For this review, take the finished solid that the model builds, in its own axes (mm). Round coordinates to 2 decimals unless told otherwise and drop trailing zeros. Loops run counter-clockwise (first coordinate to the right, second up) from the corner with the lowest first, then second, coordinate; pieces in that order, holes last. Notation, with made-up numbers: (-30.75, 60) -> (-11.75, 60) arc R29 ccw to (-11.75, 96) -> close; hole circle Ø5 at (65, -16.5). An arc over 180 degrees is marked (long way). Use one line per item in the form item = value. Start each with the question number.
from build123d import *

# Parameters (mm, degrees)
SKETCH_1_W          = 271
SKETCH_1_H          = 420.5
EXTRUDE_1_DEPTH     = 4
SKETCH_2_R          = 2.1
CUT_EXTRUDE_1_DEPTH = 251.162572141
EXTRUDE_2_DEPTH     = 4
FILLET_2_R          = 10
SKETCH_7_R          = 1.6
CUT_EXTRUDE_4_DEPTH = 261.756231949
SKETCH_8_W          = 88
SKETCH_8_H          = 60
EXTRUDE_3_DEPTH     = 4
FILLET_3_R          = 10
SKETCH_9_R          = 2.1
CUT_EXTRUDE_5_DEPTH = 303.34303779
SKETCH_10_R         = 2.6
CUT_EXTRUDE_6_DEPTH = 4
SKETCH_12_W         = 271
SKETCH_12_H         = 62.828427
EXTRUDE_4_DEPTH     = 4
FILLET_4_R          = 10


with BuildPart() as part:
    # 草图1 → 凸台-拉伸1 (new body)
    with BuildSketch(Plane(origin=(0, 0, 0), x_dir=(1, 0, 0), z_dir=(0, 1, 0))):
        Rectangle(SKETCH_1_W, SKETCH_1_H)
    extrude(amount=EXTRUDE_1_DEPTH)

    # 草图2 → 切除-拉伸1 (cut, through all)
    with BuildSketch(Plane(origin=(0, 4, 0), x_dir=(1, 0, 0), z_dir=(0, 1, 0))):
        with Locations(Location((112, 195.75, 0), (0, 0, 270))):
            Circle(SKETCH_2_R)
        with Locations(Location((128, 195.75, 0), (0, 0, 270))):
            Circle(SKETCH_2_R)
        with Locations(Location((112, 163.75, 0), (0, 0, 270))):
            Circle(SKETCH_2_R)
        with Locations(Location((128, 163.75, 0), (0, 0, 270))):
            Circle(SKETCH_2_R)
        with Locations(Location((-128, 163.75, 0), (0, 0, 90))):
            Circle(SKETCH_2_R)
        with Locations(Location((-112, 163.75, 0), (0, 0, 90))):
            Circle(SKETCH_2_R)
        with Locations(Location((-128, 195.75, 0), (0, 0, 90))):
            Circle(SKETCH_2_R)
        with Locations(Location((-112, 195.75, 0), (0, 0, 90))):
            Circle(SKETCH_2_R)
        with Locations(Location((128, -124.25, 0), (0, 0, 270))):
            Circle(SKETCH_2_R)
        with Locations(Location((112, -124.25, 0), (0, 0, 270))):
            Circle(SKETCH_2_R)
        with Locations(Location((128, -156.25, 0), (0, 0, 270))):
            Circle(SKETCH_2_R)
        with Locations(Location((112, -156.25, 0), (0, 0, 270))):
            Circle(SKETCH_2_R)
        with Locations(Location((-112, -156.25, 0), (0, 0, 90))):
            Circle(SKETCH_2_R)
        with Locations(Location((-128, -156.25, 0), (0, 0, 90))):
            Circle(SKETCH_2_R)
        with Locations(Location((-112, -124.25, 0), (0, 0, 90))):
            Circle(SKETCH_2_R)
        with Locations(Location((-128, -124.25, 0), (0, 0, 90))):
            Circle(SKETCH_2_R)
    extrude(amount=-CUT_EXTRUDE_1_DEPTH, mode=Mode.SUBTRACT)

    # 草图3 → 凸台-拉伸2 (add)
    with BuildSketch(Plane(origin=(0, 4, 0), x_dir=(1, 0, 0), z_dir=(0, 1, 0))):
        Polygon((-135.5, -215), (-135.5, -210.25), (135.5, -210.25), (135.5, -215), (135.5, -222.75), (102, -222.75), (-102, -222.75), (-135.5, -222.75), align=None)
    extrude(amount=-EXTRUDE_2_DEPTH)

    # 圆角2
    fillet_2_edges = [part.edges().sort_by_distance(p)[0] for p in [
        (-135.5, 2, -210.25),
        (135.5, 2, -210.25),
    ]]
    fillet(fillet_2_edges, radius=FILLET_2_R)

    # 草图7 → 切除-拉伸4 (cut, through all)
    with BuildSketch(Plane.XZ):
        with Locations(Location((-51.5, -131.75, 0), (0, 0, 270))):
            Circle(SKETCH_7_R)
        with Locations(Location((-35.5, -131.75, 0), (0, 0, 270))):
            Circle(SKETCH_7_R)
        with Locations(Location((35.5, -131.75, 0), (0, 0, 90))):
            Circle(SKETCH_7_R)
        with Locations(Location((51.5, -131.75, 0), (0, 0, 90))):
            Circle(SKETCH_7_R)
        with Locations(Location((-51.5, 92.25, 0), (0, 0, 270))):
            Circle(SKETCH_7_R)
        with Locations(Location((-35.5, 92.25, 0), (0, 0, 270))):
            Circle(SKETCH_7_R)
        with Locations(Location((35.5, 92.25, 0), (0, 0, 90))):
            Circle(SKETCH_7_R)
        with Locations(Location((51.5, 92.25, 0), (0, 0, 90))):
            Circle(SKETCH_7_R)
        with Locations(Location((-35.5, -27.75, 0), (0, 0, 270))):
            Circle(SKETCH_7_R)
        with Locations(Location((-35.5, -11.75, 0), (0, 0, 270))):
            Circle(SKETCH_7_R)
        with Locations(Location((35.5, -11.75, 0), (0, 0, 90))):
            Circle(SKETCH_7_R)
        with Locations(Location((35.5, -27.75, 0), (0, 0, 90))):
            Circle(SKETCH_7_R)
    extrude(amount=-CUT_EXTRUDE_4_DEPTH, mode=Mode.SUBTRACT)

    # 草图8 → 凸台-拉伸3 (add)
    with BuildSketch(Plane.XZ):
        with Locations((0, -240.25)):
            Rectangle(SKETCH_8_W, SKETCH_8_H)
    extrude(amount=-EXTRUDE_3_DEPTH)

    # 圆角3
    fillet_3_edges = [part.edges().sort_by_distance(p)[0] for p in [
        (44, 2, -270.25),
        (-44, 2, -270.25),
    ]]
    fillet(fillet_3_edges, radius=FILLET_3_R)

    # 草图9 → 切除-拉伸5 (cut, through all)
    with BuildSketch(Plane.XZ):
        with Locations(Location((-8, 157.35, 0), (0, 0, 270))):
            Circle(SKETCH_9_R)
        with Locations(Location((8, 157.35, 0), (0, 0, 270))):
            Circle(SKETCH_9_R)
        with Locations(Location((-8, 141.35, 0), (0, 0, 270))):
            Circle(SKETCH_9_R)
        with Locations(Location((8, 141.35, 0), (0, 0, 270))):
            Circle(SKETCH_9_R)
    extrude(amount=-CUT_EXTRUDE_5_DEPTH, mode=Mode.SUBTRACT)

    # 草图10 → 切除-拉伸6 (cut)
    with BuildSketch(Plane.XZ):
        with Locations(Location((-112, 208.75, 0), (0, 0, 270))):
            Circle(SKETCH_10_R)
        with Locations(Location((-112, 176.75, 0), (0, 0, 270))):
            Circle(SKETCH_10_R)
        with Locations(Location((112, 176.75, 0), (0, 0, 90))):
            Circle(SKETCH_10_R)
        with Locations(Location((112, 208.75, 0), (0, 0, 90))):
            Circle(SKETCH_10_R)
    extrude(amount=-CUT_EXTRUDE_6_DEPTH, mode=Mode.SUBTRACT)

    # 草图12 → 凸台-拉伸4 (add)
    with BuildSketch(Plane.XZ):
        with Locations((0, 254.1642135)):
            Rectangle(SKETCH_12_W, SKETCH_12_H)
    extrude(amount=-EXTRUDE_4_DEPTH)

    # 圆角4
    fillet_4_edges = [part.edges().sort_by_distance(p)[0] for p in [
        (44, 2, -210.25),
        (-44, 2, -210.25),
        (135.5, 2, 285.578427),
        (-135.5, 2, 285.578427),
    ]]
    fillet(fillet_4_edges, radius=FILLET_4_R)


solid = part.part
Item 1: Wall thickness on line 1 (X direction, y = 3.2, z = 124.25); line 2 (Z direction, x = -87.5, y = 1.5); line 3 (Z direction, x = -128, y = 1.6): over which ranges is each line inside the solid? List them lowest first.
Item 2: Take a section at A-A on y = 1.4. Give the number of separate pieces and of enclosed holes in the cut face, plus the area to 3 significant figures.
Item 3: Take a section at B-B on x = -99.5. Give the boundary of the cut face in (y, z).
Results:
q1.line_1 = -135.5 to -130.1, -125.9 to -114.1, -109.9 to 109.9, 114.1 to 125.9, 130.1 to 135.5
q1.line_2 = -210.25 to 285.58
q1.line_3 = -209.93 to -197.85, -193.65 to -165.85, -161.65 to 122.15, 126.35 to 154.15, 158.35 to 285.26
q2.separate_pieces = 1
q2.enclosed_holes = 36
q2.area = 139,000 mm2
q3.outline = (0, -210.25) -> (4, -210.25) -> (4, 285.58) -> (0, 285.58) -> close
